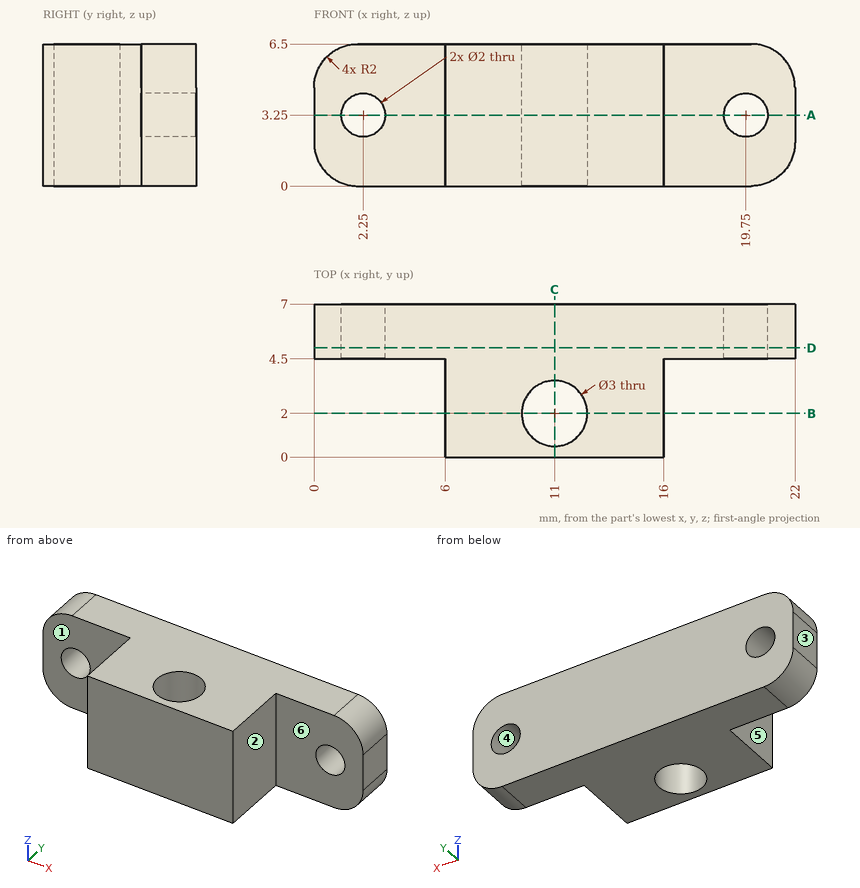
Here's the drawing with two shaded views (mm, measured from the low corner). I have some questions. A direction names the side the tool comes from. Coordinates: 2 decimals unless noted, no trailing zeros. Order: outer loops, then holes, each group sorted by start corner. A loop starts at its lowest first (then second) coordinate and runs counter-clockwise, first axis right, second up. Notation, with made-up numbers: M 64,-38.5 L 100,-38.5 A22 ccw 100,-19.5 Z; hole C 77,77.25 d3. An arc over 180 degrees is marked long. Write item = value, one per line.
(1) Suppose I cut it at C-C on x = 11. Please give me the cut outline in (y, z), plus the area to 3 significant figures.
Results are:
outline = M 0,0 L 0.5,0 L 0.5,6.5 L 0,6.5 Z; M 3.5,0 L 7,0 L 7,6.5 L 3.5,6.5 Z
area = 26.0 mm2
(2) Suppose I cut it at A-A on z = 3.25. Please give me the cut outline in (x, y).
Results are:
outline = M 0,4.5 L 1.25,4.5 L 1.25,7 L 0,7 Z; M 3.25,4.5 L 6,4.5 L 6,0 L 16,0 L 16,4.5 L 18.75,4.5 L 18.75,7 L 3.25,7 Z; M 20.75,4.5 L 22,4.5 L 22,7 L 20.75,7 Z; hole C 11,2 d3
(3) I need wall thicknesses on line 1 along X through (y, z) = (5.3, 3.25); line 2 along Z through (x, y) = (19.75, 5.2); line 3 along Y through (x, z) = (20, 2.25). Which ranges of each line are inside material? Lowest first, please. Write a range as [from, to].
Results are:
line_1 = [0, 1.25], [3.25, 18.75], [20.75, 22]
line_2 = [0, 2.25], [4.25, 6.5]
line_3 = [4.5, 7]
(4) Suppose I cut it at D-D on y = 5. Please give me the cut outline in (x, z), plus the area to 3 significant figures.
Results are:
outline = M 0,2 A2 ccw 2,0 L 20,0 A2 ccw 22,2 L 22,4.5 A2 ccw 20,6.5 L 2,6.5 A2 ccw 0,4.5 Z; hole C 2.25,3.25 d2; hole C 19.75,3.25 d2
area = 133 mm2
(5) If we mould it in two halves opening along X, with no side actions, what happens to the marked faces 4, 5 and 6? For each: pulls with the +X half, pulls with the -X half, needs draft (parallel to the pull), parting line crosses it, or undercut.
Results are:
face_4 = undercut
face_5 = pulls with the -X half
face_6 = needs draft
(6) Suppose I cut it at B-B on y = 2. Please give me the cut outline in (x, z).
Results are:
outline = M 6,0 L 9.5,0 L 9.5,6.5 L 6,6.5 Z; M 12.5,0 L 16,0 L 16,6.5 L 12.5,6.5 Z
(7) For the marked faces 1, 2 and 3, which set-ups out of +Z, -Z, +X, -X, +Y, -Y let a thin tool reach every point of the face, with its end or its side?
Results are:
face_1 = +Z, -Z, -X, -Y
face_2 = +Z, -Z, +X, -Y
face_3 = +Z, -Z, -X, +Y, -Y
(8) For pin 1 Ø2 at (y, z) = (2.5, 2) entering from -X; pin 2 Ø3 at (x, z) = (19.75, 3.25) entering from -Y, each with a flat end and sliding along its axis, tell me the tip position at first contact or that it passes through.
Results are:
pin_1 = 6
pin_2 = 4.5
